Work out the finished part from the listing and answer in its coordinate system (mm). A direction names the side the tool comes from. Give positions to 0.01 mm unless a question says otherwise; leave off trailing zeros. Order: outer loops, then holes, each group sorted by start corner. A loop starts at its lowest first (then second) coordinate and runs counter-clockwise, first axis right, second up. Notation, with made-up numbers: (47, -17) -> (61, -17) arc R15 ccw to (61, 11) -> close; hole circle Ø6 at (-6.5, 20). An arc over 180 degrees is marked (long way). Answer as CSV lines item,"result". Start each with the question number.
1. A cutting plane is placed at A-A (x = 0). Give the vertices of the cut face in (y, z) (3 decimals).
2. For a pull along Z with two mould halves and no side action, classify faces 1 (the cylindrical face through (-7.86, 16.79, -1.5)), 2 (the flat face through (3, 13.9, 0)), 3 (the flat face through (-4, 6.49, 7)), 4 (the flat face through (-6.541, 15.604, -0.474)) as released by +Z, released by -Z, zero draft, split by the parting line, or undercut.
3. For faces 5 (the flat face through (-3.53, 15.34, 7.04)), 6 (the flat face through (4, 0.5, -4)), 7 (the flat face through (-4, 6.49, -7)), 8 (the flat face through (-3.1, 11.77, 5.2)), 9 (the flat face through (4.333, 15.339, 6.575)), determine the directions among +Z, -Z, +X, -X, +Y, -Y from which every point of the face is accessible in a straight line to the end or side of a thin tool.
4. Find the intervals of material crossed by L1, parallel to Z at x = 0, y = 14.3 (3 decimals); L2, parallel to Y at x = 2, z = -3; L3, parallel to Z at x = 0.25, y = 5.5, in increasing order.
5. Flat-ended cylindrical pins translate along their axes: pin 1 (0.6 mm diameter, centred on x = -2.5, z = -5, fed in from +Y); pin 2 (0.5 mm diameter, centred on x = 0.5, z = 6.5, fed in from +Y); pin 3 (0.6 mm diameter, centred on x = 3, y = 15.5, fed in from +Z). Find the tip coordinate at first contact, or state that the pin passes through.
6. A cutting plane is placed at C-C (z = -2.92). Give the vertices of the cut face in (x, y).
from build123d import *

# Parameters (mm, degrees)
SKETCH1_R               = 6.815
BOSS_EXTRUDE1_DEPTH     = 6.49
BOSS_EXTRUDE2_DEPTH     = 8.53
BOSS_EXTRUDE3_DEPTH     = 10
CIRPATTERN1_COUNT       = 6
SKETCH4_R               = 10.914422046
SKETCH4_R_2             = 8.94
CUT_EXTRUDE1_DEPTH      = 18
CUT_EXTRUDE2_DEPTH      = 18
CUT_EXTRUDE4_DEPTH      = 11.305565513
CIRPATTERN2_COUNT       = 6
SKETCH8_R               = 2.625
CUT_EXTRUDE5_DEPTH      = 2.775565513
CUT_EXTRUDE5_DEPTH_BACK = 16.02
SKETCH9_R               = 5.84
CUT_EXTRUDE6_DEPTH      = 13.9
BOSS_EXTRUDE4_DEPTH     = 13.9
CIRPATTERN3_COUNT       = 3
BOSS_EXTRUDE5_DEPTH     = 13.4
CIRPATTERN4_COUNT       = 3
SKETCH12_R              = 0.96
CUT_EXTRUDE7_DEPTH      = 3.25


with BuildPart() as part:
    # Sketch1 → Boss-Extrude1 (new body)
    with BuildSketch(Plane(origin=(0, 0, 0), x_dir=(1, 0, 0), z_dir=(0, 1, 0))):
        Circle(SKETCH1_R)
    extrude(amount=BOSS_EXTRUDE1_DEPTH)

    # Sketch2 → Boss-Extrude2 (add)
    with BuildSketch(Plane(origin=(0, 6.49, 0), x_dir=(1, 0, 0), z_dir=(0, 1, 0))):
        Polygon((3.4075, 5.901963127), (-3.4075, 5.901963127), (-6.815, 0), (-3.4075, -5.901963127), (3.4075, -5.901963127), (6.815, 0), align=None)
    extrude(amount=BOSS_EXTRUDE2_DEPTH)

    # Sketch3 → Boss-Extrude3 (add)
    with BuildSketch(Plane(origin=(0, 0, 0), x_dir=(0, 0, -1), z_dir=(1, 0, 0))):
        with BuildLine():
            Line((-2.6, 6.49), (2.6, 6.49))
            Line((2.6, 6.49), (2.6, 13.49))
            Line((2.6, 13.49), (-0.934676019, 16.550017775))
            ThreePointArc((-0.934676019, 16.550017775), (-2.011804271, 16.704512725), (-2.6, 15.789034847))
            Line((-2.6, 15.789034847), (-2.6, 13.49))
            Line((-2.6, 13.49), (-2.6, 6.49))
        make_face()
    boss_extrude3 = extrude(amount=BOSS_EXTRUDE3_DEPTH)

    # CirPattern1: Boss-Extrude3 ×6 about axis
    cirpattern1_axis = Axis((0, 0, 0), (0, 1, 0))
    for i in range(1, CIRPATTERN1_COUNT):
        add(boss_extrude3.rotate(cirpattern1_axis, i * 360 / CIRPATTERN1_COUNT))

    # Sketch4 → Cut-Extrude1 (cut)
    with BuildSketch(Plane(origin=(0, 0, 0), x_dir=(1, 0, 0), z_dir=(0, 1, 0))):
        Circle(SKETCH4_R)
        Circle(SKETCH4_R_2, mode=Mode.SUBTRACT)
    extrude(amount=CUT_EXTRUDE1_DEPTH, mode=Mode.SUBTRACT)

    # Sketch5 → Cut-Extrude2 (cut)
    with BuildSketch(Plane(origin=(0, 15.02, 0), x_dir=(1, 0, 0), z_dir=(0, 1, 0))):
        Polygon((-3.4075, 5.901963127), (-6.815, 0), (-3.4075, -5.901963127), (3.4075, -5.901963127), (6.815, 0), (3.4075, 5.901963127), align=None)
    extrude(amount=CUT_EXTRUDE2_DEPTH, mode=Mode.SUBTRACT)

    # Sketch7 → Cut-Extrude4 (cut, through all)
    with BuildSketch(Plane(origin=(0, 6.49, 0), x_dir=(1, 0, 0), z_dir=(0, 1, 0))):
        Polygon((-6.213841686, -1.041236743), (-8.553572353, -2.6), (-5.3138893, -2.6), align=None)
        Polygon((-8.553572353, 2.6), (-6.275364549, 0.934676019), (-5.3138893, 2.6), align=None)
    cut_extrude4 = extrude(amount=CUT_EXTRUDE4_DEPTH, mode=Mode.SUBTRACT)

    # CirPattern2: Cut-Extrude4 ×6 about axis
    cirpattern2_axis = Axis((0, 0, 0), (0, 1, 0))
    for i in range(1, CIRPATTERN2_COUNT):
        add(cut_extrude4.rotate(cirpattern2_axis, i * 360 / CIRPATTERN2_COUNT), mode=Mode.SUBTRACT)

    # Sketch8 → Cut-Extrude5 (cut, two sides)
    with BuildSketch(Plane(origin=(0, 15.02, 0), x_dir=(1, 0, 0), z_dir=(0, 1, 0))) as cut_extrude5_sk:
        Circle(SKETCH8_R)
    extrude(amount=CUT_EXTRUDE5_DEPTH, mode=Mode.SUBTRACT)
    extrude(cut_extrude5_sk.sketch, amount=-CUT_EXTRUDE5_DEPTH_BACK, mode=Mode.SUBTRACT)

    # Sketch9 → Cut-Extrude6 (cut)
    with BuildSketch(Plane(origin=(0, 0, 0), x_dir=(-1, 0, 0), z_dir=(0, -1, 0))):
        Circle(SKETCH9_R)
    extrude(amount=-CUT_EXTRUDE6_DEPTH, mode=Mode.SUBTRACT)

    # Sketch10 → Boss-Extrude4 (add)
    with BuildSketch(Plane(origin=(0, 0, 0), x_dir=(1, 0, 0), z_dir=(0, 1, 0))):
        with BuildLine():
            Line((-0.790866214, -5.84), (0.790866214, -5.84))
            ThreePointArc((0.790866214, -5.84), (0, -5.049133786), (-0.790866214, -5.84))
        make_face()
    boss_extrude4 = extrude(amount=BOSS_EXTRUDE4_DEPTH)

    # CirPattern3: Boss-Extrude4 ×3 about axis
    cirpattern3_axis = Axis((0, 0, 0), (0, 1, 0))
    for i in range(1, CIRPATTERN3_COUNT):
        add(boss_extrude4.rotate(cirpattern3_axis, i * 360 / CIRPATTERN3_COUNT))

    # Sketch11 → Boss-Extrude5 (add)
    with BuildSketch(Plane.XZ.offset(-13.9)):
        Polygon((1.104876589, 5.753522427), (0.982953313, 5.335499767), (1.686743969, 5.130227492), (1.811594174, 5.558285339), align=None)
    boss_extrude5 = extrude(amount=BOSS_EXTRUDE5_DEPTH)

    # CirPattern4: Boss-Extrude5 ×3 about axis
    cirpattern4_axis = Axis((0, 0, 0), (0, 1, 0))
    for i in range(1, CIRPATTERN4_COUNT):
        add(boss_extrude5.rotate(cirpattern4_axis, i * 360 / CIRPATTERN4_COUNT))

    # Sketch12 → Cut-Extrude7 (cut)
    with BuildSketch(Plane(origin=(0, 15.02, 0), x_dir=(1, 0, 0), z_dir=(0, 1, 0))):
        with Locations((-2.714264925, -4.702681498)):
            Circle(SKETCH12_R)
        with Locations((-2.714679677, 4.701963127)):
            Circle(SKETCH12_R)
        with Locations((5.429359354, 0)):
            Circle(SKETCH12_R)
    extrude(amount=-CUT_EXTRUDE7_DEPTH, mode=Mode.SUBTRACT)


solid = part.part
Answer sheet:
1,outline,"(0, -6.815) -> (6.49, -6.815) -> (6.49, -5.902) -> (15.02, -5.902) -> (15.02, -2.625) -> (13.9, -2.625) -> (13.9, -5.84) -> (0, -5.84) -> close; (0, 5.049) -> (13.9, 5.049) -> (13.9, 2.625) -> (15.02, 2.625) -> (15.02, 5.902) -> (6.49, 5.902) -> (6.49, 6.815) -> (0, 6.815) -> close"
2,face 1,"split by the parting line"
2,face 2,"undercut"
2,face 3,"zero draft"
2,face 4,"undercut"
3,face 5,"+Z, +Y"
3,face 6,"-Y"
3,face 7,"-Z, -X, -Y"
3,face 8,"+Y"
3,face 9,"+X, +Y"
4,L1,"z = -5.902 to -2.625, 2.625 to 5.902"
4,L2,"y = 13.9 to 15.02"
4,L3,"z = -6.81 to -5.83, 5.09 to 6.81"
5,pin 1,"stops at y = 11.77"
5,pin 2,"stops at y = 6.49"
5,pin 3,"stops at z = 8.52"
6,outline,"(-6.16, 0) -> (-4.27, 0) -> (-4.27, 13.9) -> (4.27, 13.9) -> (4.27, 0) -> (6.16, 0) -> (6.16, 6.49) -> (5.13, 6.49) -> (5.13, 15.02) -> (-5.13, 15.02) -> (-5.13, 6.49) -> (-6.16, 6.49) -> close"
